```python
from build123d import *

# Parameters (mm, degrees)
SKETCH1_W           = 30
SKETCH1_H           = 30
BOSS_EXTRUDE1_DEPTH = 10
SKETCH2_R           = 9.6
SKETCH2_R_2         = 9.55
CUT_EXTRUDE1_DEPTH  = 7
SKETCH3_R           = 4
CUT_EXTRUDE2_DEPTH  = 7
SKETCH4_R           = 2
CUT_EXTRUDE3_DEPTH  = 10
CIRPATTERN1_COUNT   = 4
SKETCH5_W           = 30
SKETCH5_H           = 10
BOSS_EXTRUDE2_DEPTH = 60
SKETCH6_W           = 30
SKETCH6_H           = 50
BOSS_EXTRUDE3_DEPTH = 5


with BuildPart() as part:
    # Sketch1 → Boss-Extrude1 (new body)
    with BuildSketch(Plane(origin=(0, 0, 0), x_dir=(1, 0, 0), z_dir=(0, 1, 0))):
        Rectangle(SKETCH1_W, SKETCH1_H)
    extrude(amount=BOSS_EXTRUDE1_DEPTH)

    # Sketch2 → Cut-Extrude1 (cut)
    with BuildSketch(Plane(origin=(0, 10, 0), x_dir=(1, 0, 0), z_dir=(0, 1, 0))):
        Circle(SKETCH2_R)
        Circle(SKETCH2_R_2, mode=Mode.SUBTRACT)
    extrude(amount=-CUT_EXTRUDE1_DEPTH, mode=Mode.SUBTRACT)

    # Sketch3 → Cut-Extrude2 (cut)
    with BuildSketch(Plane(origin=(0, 10, 0), x_dir=(1, 0, 0), z_dir=(0, 1, 0))):
        Circle(SKETCH3_R)
    extrude(amount=-CUT_EXTRUDE2_DEPTH, mode=Mode.SUBTRACT)

    # Sketch4 → Cut-Extrude3 (cut)
    with BuildSketch(Plane(origin=(0, 10, 0), x_dir=(1, 0, 0), z_dir=(0, 1, 0))):
        with Locations((10.792349727, 10.987509758)):
            Circle(SKETCH4_R)
    cut_extrude3 = extrude(amount=-CUT_EXTRUDE3_DEPTH, mode=Mode.SUBTRACT)

    # CirPattern1: Cut-Extrude3 ×4 about axis
    cirpattern1_axis = Axis((0, 0, 0), (0, 1, 0))
    for i in range(1, CIRPATTERN1_COUNT):
        add(cut_extrude3.rotate(cirpattern1_axis, i * 360 / CIRPATTERN1_COUNT), mode=Mode.SUBTRACT)

    # Sketch5 → Boss-Extrude2 (add)
    with BuildSketch(Plane(origin=(0, 0, -15), x_dir=(-1, 0, 0), z_dir=(0, 0, -1))):
        with Locations((0, 5)):
            Rectangle(SKETCH5_W, SKETCH5_H)
    extrude(amount=BOSS_EXTRUDE2_DEPTH)

    # Sketch6 → Boss-Extrude3 (add)
    with BuildSketch(Plane(origin=(0, 0, -75), x_dir=(-1, 0, 0), z_dir=(0, 0, -1))):
        with Locations((0.023044467, 5)):
            Rectangle(SKETCH6_W, SKETCH6_H)
    extrude(amount=-BOSS_EXTRUDE3_DEPTH)


solid = part.part
```
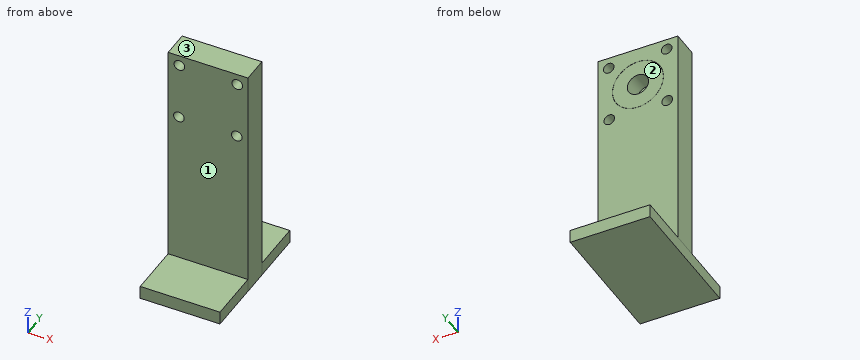
Input: part model. Units: mm. Frame: model coordinates. Face numbers are marked on the shaded views. A direction names the side the tool comes from. Coordinates: 2 decimals unless noted, no trailing zeros. Loops run counter-clockwise (first coordinate to the right, second up) from the corner with the lowest first, then second, coordinate; pieces in that order, holes last.
Q1. Section C-C, the plane y = -6.5. Return the cut outline in (x, z).
Results are:
outline: (-15.02, -75) - (14.98, -75) - (14.98, -70) - (-15.02, -70) - close
Q2. Line query: line 1 along Z through (x, y) = (12, 9.5); line 2 along Y through (x, z) = (11, -54); line 3 along Z through (x, y) = (-0.5, -9). Output: solid intervals per line, ascending.
Results are:
line 1: z = -75 to -12.58, -9.39 to 9.07, 12.52 to 15
line 2: y = 0 to 10
line 3: z = -75 to -70
Q3. Section A-A, the plane x = 0. Return the cut outline in (y, z), and give its area (3 significant figures).
Results are:
outline: (-20, -75) - (30, -75) - (30, -70) - (10, -70) - (10, -9.6) - (3, -9.6) - (3, -9.55) - (10, -9.55) - (10, -4) - (3, -4) - (3, 4) - (10, 4) - (10, 9.55) - (3, 9.55) - (3, 9.6) - (10, 9.6) - (10, 15) - (0, 15) - (0, -70) - (-20, -70) - close
area: 1,040 mm2
Q4. Section B-B, the plane z = 0. Return the cut outline in (x, y).
Results are:
outline: (-15, 0) - (15, 0) - (15, 10) - (9.6, 10) - (9.6, 3) - (9.55, 3) - (9.55, 10) - (4, 10) - (4, 3) - (-4, 3) - (-4, 10) - (-9.55, 10) - (-9.55, 3) - (-9.6, 3) - (-9.6, 10) - (-15, 10) - close
Q5. Section D-D, the plane x = -6. Return the cut outline in (y, z).
Results are:
outline: (-20, -75) - (30, -75) - (30, -70) - (10, -70) - (10, -7.49) - (3, -7.49) - (3, -7.43) - (10, -7.43) - (10, 7.43) - (3, 7.43) - (3, 7.49) - (10, 7.49) - (10, 15) - (0, 15) - (0, -70) - (-20, -70) - close
Q6. Contact query for flat-ended pins moving along their axis: pin 1 (4 mm diameter, centred on x = 10, z = -44, fed in from -Y); pin 2 (2 mm diameter, centred on x = -7, y = -14, fed in from +Z); pin 3 (9 mm diameter, centred on x = 0, z = 0, fed in from +Y). Output: stop coordinate, or through.
Results are:
pin 1: stops at y = 0
pin 2: stops at z = -70
pin 3: stops at y = 10
Q7. Set-up query: the marked faces 1, 2 and 3. Return all of +Z, -Z, +X, -X, +Y, -Y with unobstructed straight access to the full face (end or side cutting, diameter ignored); none if empty.
Results are:
face 1: +Z, +X, -X, -Y
face 2: +Z, +X, -X, +Y
face 3: +Z, +X, -X, +Y, -Y
